```python
from build123d import *

# Parameters (mm, degrees)
SKETCH1_W           = 152.4
SKETCH1_H           = 203.2
BOSS_EXTRUDE2_DEPTH = 6.35
SKETCH2_R           = 1.5
CUT_EXTRUDE1_DEPTH  = 128.158650905
SKETCH3_R           = 1.5
CUT_EXTRUDE2_DEPTH  = 128.158650905
SKETCH4_R           = 1.5
CUT_EXTRUDE3_DEPTH  = 128.158650905
SKETCH5_R           = 44.45
BOSS_EXTRUDE3_DEPTH = 114.3
SHELL1_START        = 2.54
SHELL1_OUTLINE_R    = 41.91
SHELL1_DEPTH        = 118.11
SHELL1_2_OUTLINE_R  = 41.91
SHELL1_2_DEPTH      = 1.27
SKETCH6_R           = 38.1
CUT_EXTRUDE4_DEPTH  = 5.08
SKETCH7_W           = 17.78
SKETCH7_H           = 18.673076246
CUT_EXTRUDE5_DEPTH  = 5.08
SKETCH8_W           = 19.05
SKETCH8_H           = 19.05
CUT_EXTRUDE6_DEPTH  = 171.861025398
SKETCH9_W           = 27.94
SKETCH9_H           = 27.94
CUT_EXTRUDE7_DEPTH  = 4.318
SKETCH10_W          = 12.7
SKETCH10_H          = 3.048
CUT_EXTRUDE9_DEPTH  = 174.779256311
SKETCH12_W          = 25.4
SKETCH12_H          = 67.31
BOSS_EXTRUDE5_DEPTH = 55.88
SHELL3_START        = 39.044015943
SHELL3_OUTLINE_W    = 52.07
SHELL3_OUTLINE_H    = 57.15
SHELL3_DEPTH        = 20.32
SKETCH13_W          = 20.303180985
SKETCH13_H          = 25.4
CUT_EXTRUDE10_DEPTH = 55.88
SKETCH17_W          = 25.4
SKETCH17_H          = 44.45
CUT_EXTRUDE11_DEPTH = 3.048
SKETCH18_W          = 24.931380967
SKETCH18_H          = 13.519409137
CUT_EXTRUDE12_DEPTH = 10.668
SKETCH19_W          = 25.074639176
SKETCH19_H          = 10.629198189
CUT_EXTRUDE13_DEPTH = 10.668
SKETCH20_W          = 12.7
SKETCH20_H          = 12.7
CUT_EXTRUDE14_DEPTH = 3.048
SKETCH22_W          = 2.266473324
SKETCH22_H          = 12.172894029
CUT_EXTRUDE15_DEPTH = 5.08
SKETCH23_W          = 2.681145579
SKETCH23_H          = 12.278390502
CUT_EXTRUDE16_DEPTH = 5.08


# Read off the part's stored shape, not the designer's step: Shell1, Shell3
with BuildPart() as part:
    # Sketch1 → Boss-Extrude2 (new body)
    with BuildSketch(Plane(origin=(0, 0, 0), x_dir=(1, 0, 0), z_dir=(0, 1, 0))):
        Rectangle(SKETCH1_W, SKETCH1_H)
    extrude(amount=BOSS_EXTRUDE2_DEPTH)

    # Sketch2 → Cut-Extrude1 (cut, through all)
    with BuildSketch(Plane(origin=(0, 6.35, 0), x_dir=(1, 0, 0), z_dir=(0, 1, 0))):
        with Locations(Location((-69.85, 95.25, 0), (0, 0, 270))):
            Circle(SKETCH2_R)
    extrude(amount=-CUT_EXTRUDE1_DEPTH, mode=Mode.SUBTRACT)

    # Sketch3 → Cut-Extrude2 (cut, through all)
    with BuildSketch(Plane(origin=(0, 6.35, 0), x_dir=(1, 0, 0), z_dir=(0, 1, 0))):
        with Locations(Location((69.85, 95.25, 0), (0, 0, 270))):
            Circle(SKETCH3_R)
    extrude(amount=-CUT_EXTRUDE2_DEPTH, mode=Mode.SUBTRACT)

    # Sketch4 → Cut-Extrude3 (cut, through all)
    with BuildSketch(Plane(origin=(0, 6.35, 0), x_dir=(1, 0, 0), z_dir=(0, 1, 0))):
        with Locations(Location((69.85, -95.25, 0), (0, 0, 270))):
            Circle(SKETCH4_R)
        with Locations(Location((-69.85, -95.25, 0), (0, 0, 270))):
            Circle(SKETCH4_R)
    extrude(amount=-CUT_EXTRUDE3_DEPTH, mode=Mode.SUBTRACT)

    # Sketch5 → Boss-Extrude3 (add)
    with BuildSketch(Plane(origin=(0, 6.35, 0), x_dir=(1, 0, 0), z_dir=(0, 1, 0))):
        with Locations(Location((-29.014615541, 52.680103604, 0), (0, 0, 270))):
            Circle(SKETCH5_R)
    extrude(amount=BOSS_EXTRUDE3_DEPTH)

    # Shell1 outline → Shell1 (cut)
    with BuildSketch(Plane(origin=(0, 0, 0), x_dir=(1, 0, 0), z_dir=(0, 1, 0)).offset(SHELL1_START)):
        with Locations((-29.014615541, 52.680103604)):
            Circle(SHELL1_OUTLINE_R)
    extrude(amount=SHELL1_DEPTH, mode=Mode.SUBTRACT)

    # Shell1 2 outline → Shell1 2 (cut)
    # profile 1 of 5: a face of its own
    with BuildSketch(Plane(origin=(0, 0, 0), x_dir=(1, 0, 0), z_dir=(0, 1, 0)).offset(SHELL1_START)):
        with BuildLine():
            ThreePointArc((-68.506311048, 99.06), (-66.993288604, 92.393288604), (-73.66, 93.906311048))
            Line((-73.66, 93.906311048), (-73.66, -93.906311048))
            ThreePointArc((-73.66, -93.906311048), (-66.993288604, -92.393288604), (-68.506311048, -99.06))
            Line((-68.506311048, -99.06), (68.506311048, -99.06))
            ThreePointArc((68.506311048, -99.06), (66.993288604, -92.393288604), (73.66, -93.906311048))
            Line((73.66, -93.906311048), (73.66, 93.906311048))
            ThreePointArc((73.66, 93.906311048), (66.993288604, 92.393288604), (68.506311048, 99.06))
            Line((68.506311048, 99.06), (-68.506311048, 99.06))
        make_face()
        with Locations((-29.014615541, 52.680103604)):
            Circle(SHELL1_2_OUTLINE_R, mode=Mode.SUBTRACT)
    # profile 2 of 5: a face of its own
    with BuildSketch(Plane(origin=(0, 0, 0), x_dir=(1, 0, 0), z_dir=(0, 1, 0)).offset(SHELL1_START)):
        with BuildLine():
            ThreePointArc((-73.66, 96.593688952), (-72.706711396, 98.106711396), (-71.193688952, 99.06))
            Line((-71.193688952, 99.06), (-73.66, 99.06))
            Line((-73.66, 99.06), (-73.66, 96.593688952))
        make_face()
    # profile 3 of 5: a face of its own
    with BuildSketch(Plane(origin=(0, 0, 0), x_dir=(1, 0, 0), z_dir=(0, 1, 0)).offset(SHELL1_START)):
        with BuildLine():
            Line((73.66, 99.06), (71.193688952, 99.06))
            ThreePointArc((71.193688952, 99.06), (72.706711396, 98.106711396), (73.66, 96.593688952))
            Line((73.66, 96.593688952), (73.66, 99.06))
        make_face()
    # profile 4 of 5: a face of its own
    with BuildSketch(Plane(origin=(0, 0, 0), x_dir=(1, 0, 0), z_dir=(0, 1, 0)).offset(SHELL1_START)):
        with BuildLine():
            Line((73.66, -99.06), (73.66, -96.593688952))
            ThreePointArc((73.66, -96.593688952), (72.706711396, -98.106711396), (71.193688952, -99.06))
            Line((71.193688952, -99.06), (73.66, -99.06))
        make_face()
    # profile 5 of 5: a face of its own
    with BuildSketch(Plane(origin=(0, 0, 0), x_dir=(1, 0, 0), z_dir=(0, 1, 0)).offset(SHELL1_START)):
        with BuildLine():
            ThreePointArc((-71.193688952, -99.06), (-72.706711396, -98.106711396), (-73.66, -96.593688952))
            Line((-73.66, -96.593688952), (-73.66, -99.06))
            Line((-73.66, -99.06), (-71.193688952, -99.06))
        make_face()
    extrude(amount=SHELL1_2_DEPTH, mode=Mode.SUBTRACT)

    # Sketch6 → Cut-Extrude4 (cut)
    with BuildSketch(Plane(origin=(0, 6.35, 0), x_dir=(1, 0, 0), z_dir=(0, 1, 0))):
        with Locations(Location((-31.166979336, -58.42, 0), (0, 0, 270))):
            Circle(SKETCH6_R)
    extrude(amount=-CUT_EXTRUDE4_DEPTH, mode=Mode.SUBTRACT)

    # Sketch7 → Cut-Extrude5 (cut)
    with BuildSketch(Plane(origin=(0, 1.27, 0), x_dir=(1, 0, 0), z_dir=(0, 1, 0))):
        with Locations((-31.166979336, -96.52)):
            Rectangle(SKETCH7_W, SKETCH7_H)
    extrude(amount=CUT_EXTRUDE5_DEPTH, mode=Mode.SUBTRACT)

    # Sketch8 → Cut-Extrude6 (cut, through all)
    with BuildSketch(Plane(origin=(0, 6.35, 0), x_dir=(1, 0, 0), z_dir=(0, 1, 0))):
        with Locations((2.757472123, -2.376350246)):
            Rectangle(SKETCH8_W, SKETCH8_H)
    extrude(amount=-CUT_EXTRUDE6_DEPTH, mode=Mode.SUBTRACT)

    # Sketch9 → Cut-Extrude7 (cut)
    with BuildSketch(Plane(origin=(0, 6.35, 0), x_dir=(1, 0, 0), z_dir=(0, 1, 0))):
        with Locations((48.191649932, -74.237208762)):
            Rectangle(SKETCH9_W, SKETCH9_H)
    extrude(amount=-CUT_EXTRUDE7_DEPTH, mode=Mode.SUBTRACT)

    # Sketch10 → Cut-Extrude9 (cut, through all)
    with BuildSketch(Plane(origin=(0, 2.032, 0), x_dir=(1, 0, 0), z_dir=(0, 1, 0))):
        with Locations((48.191649932, -61.791208762)):
            Rectangle(SKETCH10_W, SKETCH10_H)
    extrude(amount=-CUT_EXTRUDE9_DEPTH, mode=Mode.SUBTRACT)

    # Sketch12 → Boss-Extrude5 (add)
    with BuildSketch(Plane(origin=(0, 6.35, 0), x_dir=(1, 0, 0), z_dir=(0, 1, 0))):
        with Locations((46.664015943, 49.057368238)):
            Rectangle(SKETCH12_W, SKETCH12_H)
    extrude(amount=BOSS_EXTRUDE5_DEPTH)

    # Shell3 outline → Shell3 (cut)
    with BuildSketch(Plane.YZ.offset(SHELL3_START)):
        with Locations((31.115, -49.057368238)):
            Rectangle(SHELL3_OUTLINE_W, SHELL3_OUTLINE_H)
    extrude(amount=SHELL3_DEPTH, mode=Mode.SUBTRACT)

    # Sketch13 → Cut-Extrude10 (cut)
    with BuildSketch(Plane(origin=(0, 5.08, 0), x_dir=(1, 0, 0), z_dir=(0, 1, 0))):
        with Locations((49.212425451, 33.146004513)):
            Rectangle(SKETCH13_W, SKETCH13_H)
    extrude(amount=-CUT_EXTRUDE10_DEPTH, mode=Mode.SUBTRACT)

    # Sketch17 → Cut-Extrude11 (cut)
    with BuildSketch(Plane(origin=(0, 6.35, 0), x_dir=(1, 0, 0), z_dir=(0, 1, 0))):
        with Locations((45.24021519, -21.500928879)):
            Rectangle(SKETCH17_W, SKETCH17_H)
    extrude(amount=-CUT_EXTRUDE11_DEPTH, mode=Mode.SUBTRACT)

    # Sketch18 → Cut-Extrude12 (cut)
    with BuildSketch(Plane(origin=(0, 2.54, 0), x_dir=(1, 0, 0), z_dir=(0, 1, 0))):
        with Locations((45.232741318, -6.278596744)):
            Rectangle(SKETCH18_W, SKETCH18_H)
    extrude(amount=-CUT_EXTRUDE12_DEPTH, mode=Mode.SUBTRACT)

    # Sketch19 → Cut-Extrude13 (cut)
    with BuildSketch(Plane(origin=(0, 2.54, 0), x_dir=(1, 0, 0), z_dir=(0, 1, 0))):
        with Locations((45.198109279, -38.227166647)):
            Rectangle(SKETCH19_W, SKETCH19_H)
    extrude(amount=-CUT_EXTRUDE13_DEPTH, mode=Mode.SUBTRACT)

    # Sketch20 → Cut-Extrude14 (cut)
    with BuildSketch(Plane(origin=(0, 6.35, 0), x_dir=(1, 0, 0), z_dir=(0, 1, 0))):
        with Locations((19.089329665, -82.100593314)):
            Rectangle(SKETCH20_W, SKETCH20_H)
    extrude(amount=-CUT_EXTRUDE14_DEPTH, mode=Mode.SUBTRACT)

    # Sketch22 → Cut-Extrude15 (cut)
    with BuildSketch(Plane(origin=(0, 2.54, 0), x_dir=(1, 0, 0), z_dir=(0, 1, 0))):
        with Locations((13.956818217, -81.881158104)):
            Rectangle(SKETCH22_W, SKETCH22_H)
    extrude(amount=-CUT_EXTRUDE15_DEPTH, mode=Mode.SUBTRACT)

    # Sketch23 → Cut-Extrude16 (cut)
    with BuildSketch(Plane(origin=(0, 2.54, 0), x_dir=(1, 0, 0), z_dir=(0, 1, 0))):
        with Locations((23.958869164, -82.026056303)):
            Rectangle(SKETCH23_W, SKETCH23_H)
    extrude(amount=-CUT_EXTRUDE16_DEPTH, mode=Mode.SUBTRACT)


solid = part.part
```
Input: part model. Units: mm. Frame: model coordinates. A direction names the side the tool comes from. Coordinates: 2 decimals unless noted, no trailing zeros. Write each loop counter-clockwise with the first axis right and the second up, starting at its lowest first coordinate (ties: lowest second). Pieces come first, ordered by that corner, then holes. Notation, with made-up numbers: (57.5, 6) -> (77.5, 6) arc R22 cw to (77.5, 42) -> close; hole circle Ø3 at (51.5, 75.25). An arc over 180 degrees is marked (long way). Answer as a JSON object with one key per item and string values.
1. First-contact query: P1, Ø2.5, axis at x = -72.5, z = 98, coming from the +Y side; P2, Ø2, axis at x = 0, y = 50.5, coming from the -Z side; P3, Ø2, axis at x = -5.5, z = -76.5, coming from the -Y side; P4, Ø8.5, axis at x = 43, z = 80.5, coming from the +Y side. Flat tips, straight axial feed; report the tip coordinate or a pass-through.
Result set:
{"P1": "stops at y = 6.35", "P2": "stops at z = -87.19", "P3": "stops at y = 0", "P4": "stops at y = 2.03"}
2. Material intervals for line 1 (X direction, y = 3, z = 95.25); line 2 (Z direction, x = -69.85, y = 2.25); line 3 (Y direction, x = 34.5, z = -30), sorted ascending. Write a range as from..to.
Result set:
{"line 1": "x = -76.2..-71.35, -68.35..-65.81, 65.81..68.35, 71.35..76.2", "line 2": "z = -101.6..-96.75, -93.75..93.75, 96.75..101.6", "line 3": "y = 0..2.54, 3.81..62.23"}
3. Section B-B on z = -33. Count the separate pieces of the cut face and the enclosed holes in it, then the cut area to 3 significant figures.
Result set:
{"separate pieces": "3", "enclosed holes": "0", "area": "1,530 mm2"}
4. Section C-C on x = -26. Return the cut outline in (y, z).
Result set:
{"outline": "(0, -101.6) -> (6.35, -101.6) -> (6.35, -97.03) -> (120.65, -97.03) -> (120.65, -94.48) -> (3.81, -94.48) -> (3.81, -99.06) -> (2.54, -99.06) -> (2.54, 20.67) -> (1.27, 20.67) -> (1.27, 101.6) -> (0, 101.6) -> close; (3.81, -10.88) -> (120.65, -10.88) -> (120.65, -8.33) -> (6.35, -8.33) -> (6.35, 20.67) -> (3.81, 20.67) -> close"}
5. Section A-A on y = 39.5. Return the cut outline in (x, z), then the cut area to 3 significant figures.
Result set:
{"outline": "circle Ø88.9 at (-29.01, -52.68); (33.96, -82.71) -> (59.36, -82.71) -> (59.36, -77.63) -> (39.04, -77.63) -> (39.04, -20.48) -> (59.36, -20.48) -> (59.36, -15.4) -> (33.96, -15.4) -> close; hole circle Ø83.82 at (-29.01, -52.68)", "area": "1,240 mm2"}
6. Mould query, pull axis X, two halves, no side actions, for faces 1 (the face through (59.364, 59, -49)), 2 (the face through (-1, 3, -101.6)), 3 (the face through (9.7, 61.41, -36.63)). Classes: released by +X, released by -X, zero draft, split by the parting line, or undercut.
Result set:
{"face 1": "released by +X", "face 2": "zero draft", "face 3": "undercut"}
7. Access query for faces 4 (the face through (-29.62, 1.91, 20.35)), 5 (the face through (46, 62.23, -50)), 6 (the face through (46, 34, -82.712)). Directions: +Z, -Z, +X, -X, +Y, -Y. A direction counts if a zero-diameter tool reaches every point of the face in a straight line with its end or side. Return the directions, or none.
Result set:
{"face 4": "+Y", "face 5": "+Z, -Z, +X, +Y", "face 6": "-Z, +X, +Y"}
